from build123d import *

# Parameters (mm, degrees)
F0_W      = 210.82
F0_H      = 50.8
F1_DEPTH  = 12.7
F3_DEPTH  = 10.16
F4_DEPTH  = 3.175
F6_DEPTH  = 210.82
F7_DEPTH  = 5.5118
F8_SIZE2  = 5.499251
F8_SIZE   = 9.52499
F9_R      = 1.4605
F10_DEPTH = 9.525


# Not quite as in the source:
# - a fillet or chamfer is up to 0.001 mm smaller than in the source, because OpenCascade refuses the exact size


with BuildPart() as f1:
    # F0 (on Top) → F1 (new body)
    with BuildSketch(Plane.XY):
        with Locations((105.41, 25.4)):
            Rectangle(F0_W, F0_H)
    extrude(amount=F1_DEPTH)

    # F2 (on face) → F3 (cut)
    with BuildSketch(Plane.XY.offset(12.7)):
        with BuildLine():
            ThreePointArc((8.3320384182, 43.7379615818), (6.2559880613, 44.1509136731), (5.08, 42.3909231637))
            Line((5.08, 42.3909231637), (5.08, 8.4090768363))
            ThreePointArc((5.08, 8.4090768363), (6.2559880613, 6.6490863269), (8.3320384182, 7.0620384182))
            Line((8.3320384182, 7.0620384182), (25.3229615818, 24.0529615818))
            ThreePointArc((25.3229615818, 24.0529615818), (25.8809231637, 25.4), (25.3229615818, 26.7470384182))
            Line((25.3229615818, 26.7470384182), (8.3320384182, 43.7379615818))
        make_face()
        with BuildLine():
            Line((50.0879615818, 43.7379615818), (33.0970384182, 26.7470384182))
            ThreePointArc((33.0970384182, 26.7470384182), (32.5390768363, 25.4), (33.0970384182, 24.0529615818))
            Line((33.0970384182, 24.0529615818), (50.0879615818, 7.0620384182))
            ThreePointArc((50.0879615818, 7.0620384182), (52.1640119387, 6.6490863269), (53.34, 8.4090768363))
            Line((53.34, 8.4090768363), (53.34, 42.3909231637))
            ThreePointArc((53.34, 42.3909231637), (52.1640119387, 44.1509136731), (50.0879615818, 43.7379615818))
        make_face()
        with BuildLine():
            ThreePointArc((60.4020384182, 43.7379615818), (58.3259880613, 44.1509136731), (57.15, 42.3909231637))
            Line((57.15, 42.3909231637), (57.15, 8.4090768363))
            ThreePointArc((57.15, 8.4090768363), (58.3259880613, 6.6490863269), (60.4020384182, 7.0620384182))
            Line((60.4020384182, 7.0620384182), (77.3929615818, 24.0529615818))
            ThreePointArc((77.3929615818, 24.0529615818), (77.9509231637, 25.4), (77.3929615818, 26.7470384182))
            Line((77.3929615818, 26.7470384182), (60.4020384182, 43.7379615818))
        make_face()
        with BuildLine():
            Line((104.14, 8.4090768363), (104.14, 42.3909231637))
            ThreePointArc((104.14, 42.3909231637), (102.9640119387, 44.1509136731), (100.8879615818, 43.7379615818))
            Line((100.8879615818, 43.7379615818), (83.8970384182, 26.7470384182))
            ThreePointArc((83.8970384182, 26.7470384182), (83.3390768363, 25.4), (83.8970384182, 24.0529615818))
            Line((83.8970384182, 24.0529615818), (100.8879615818, 7.0620384182))
            ThreePointArc((100.8879615818, 7.0620384182), (102.9640119387, 6.6490863269), (104.14, 8.4090768363))
        make_face()
        with BuildLine():
            ThreePointArc((111.2020384182, 43.7379615818), (109.1259880613, 44.1509136731), (107.95, 42.3909231637))
            Line((107.95, 42.3909231637), (107.95, 8.4090768363))
            ThreePointArc((107.95, 8.4090768363), (109.1259880613, 6.6490863269), (111.2020384182, 7.0620384182))
            Line((111.2020384182, 7.0620384182), (128.1929615818, 24.0529615818))
            ThreePointArc((128.1929615818, 24.0529615818), (128.7509231637, 25.4), (128.1929615818, 26.7470384182))
            Line((128.1929615818, 26.7470384182), (111.2020384182, 43.7379615818))
        make_face()
        with BuildLine():
            Line((154.94, 8.4090768363), (154.94, 42.3909231637))
            ThreePointArc((154.94, 42.3909231637), (153.7640119387, 44.1509136731), (151.6879615818, 43.7379615818))
            Line((151.6879615818, 43.7379615818), (134.6970384182, 26.7470384182))
            ThreePointArc((134.6970384182, 26.7470384182), (134.1390768363, 25.4), (134.6970384182, 24.0529615818))
            Line((134.6970384182, 24.0529615818), (151.6879615818, 7.0620384182))
            ThreePointArc((151.6879615818, 7.0620384182), (153.7640119387, 6.6490863269), (154.94, 8.4090768363))
        make_face()
        with BuildLine():
            ThreePointArc((162.0020384182, 43.7379615818), (159.9259880613, 44.1509136731), (158.75, 42.3909231637))
            Line((158.75, 42.3909231637), (158.75, 8.4090768363))
            ThreePointArc((158.75, 8.4090768363), (159.9259880613, 6.6490863269), (162.0020384182, 7.0620384182))
            Line((162.0020384182, 7.0620384182), (178.9929615818, 24.0529615818))
            ThreePointArc((178.9929615818, 24.0529615818), (179.5509231637, 25.4), (178.9929615818, 26.7470384182))
            Line((178.9929615818, 26.7470384182), (162.0020384182, 43.7379615818))
        make_face()
        with BuildLine():
            Line((205.74, 8.4090768363), (205.74, 42.3909231637))
            ThreePointArc((205.74, 42.3909231637), (204.5640119387, 44.1509136731), (202.4879615818, 43.7379615818))
            Line((202.4879615818, 43.7379615818), (185.4970384182, 26.7470384182))
            ThreePointArc((185.4970384182, 26.7470384182), (184.9390768363, 25.4), (185.4970384182, 24.0529615818))
            Line((185.4970384182, 24.0529615818), (202.4879615818, 7.0620384182))
            ThreePointArc((202.4879615818, 7.0620384182), (204.5640119387, 6.6490863269), (205.74, 8.4090768363))
        make_face()
        with BuildLine():
            Line((44.9309231637, 46.99), (13.4890768363, 46.99))
            ThreePointArc((13.4890768363, 46.99), (11.7290863269, 45.8140119387), (12.1420384182, 43.7379615818))
            Line((12.1420384182, 43.7379615818), (27.8629615818, 28.0170384182))
            ThreePointArc((27.8629615818, 28.0170384182), (29.21, 27.4590768363), (30.5570384182, 28.0170384182))
            Line((30.5570384182, 28.0170384182), (46.2779615818, 43.7379615818))
            ThreePointArc((46.2779615818, 43.7379615818), (46.6909136731, 45.8140119387), (44.9309231637, 46.99))
        make_face()
        with BuildLine():
            ThreePointArc((12.1420384182, 7.0620384182), (11.7290863269, 4.9859880613), (13.4890768363, 3.81))
            Line((13.4890768363, 3.81), (44.9309231637, 3.81))
            ThreePointArc((44.9309231637, 3.81), (46.6909136731, 4.9859880613), (46.2779615818, 7.0620384182))
            Line((46.2779615818, 7.0620384182), (30.5570384182, 22.7829615818))
            ThreePointArc((30.5570384182, 22.7829615818), (29.21, 23.3409231637), (27.8629615818, 22.7829615818))
            Line((27.8629615818, 22.7829615818), (12.1420384182, 7.0620384182))
        make_face()
        with BuildLine():
            Line((95.7309231637, 46.99), (65.5590768363, 46.99))
            ThreePointArc((65.5590768363, 46.99), (63.7990863269, 45.8140119387), (64.2120384182, 43.7379615818))
            Line((64.2120384182, 43.7379615818), (79.2979615818, 28.6520384182))
            ThreePointArc((79.2979615818, 28.6520384182), (80.645, 28.0940768363), (81.9920384182, 28.6520384182))
            Line((81.9920384182, 28.6520384182), (97.0779615818, 43.7379615818))
            ThreePointArc((97.0779615818, 43.7379615818), (97.4909136731, 45.8140119387), (95.7309231637, 46.99))
        make_face()
        with BuildLine():
            ThreePointArc((64.2120384182, 7.0620384182), (63.7990863269, 4.9859880613), (65.5590768363, 3.81))
            Line((65.5590768363, 3.81), (95.7309231637, 3.81))
            ThreePointArc((95.7309231637, 3.81), (97.4909136731, 4.9859880613), (97.0779615818, 7.0620384182))
            Line((97.0779615818, 7.0620384182), (81.9920384182, 22.1479615818))
            ThreePointArc((81.9920384182, 22.1479615818), (80.645, 22.7059231637), (79.2979615818, 22.1479615818))
            Line((79.2979615818, 22.1479615818), (64.2120384182, 7.0620384182))
        make_face()
        with BuildLine():
            Line((146.5309231637, 46.99), (116.3590768363, 46.99))
            ThreePointArc((116.3590768363, 46.99), (114.5990863269, 45.8140119387), (115.0120384182, 43.7379615818))
            Line((115.0120384182, 43.7379615818), (130.0979615818, 28.6520384182))
            ThreePointArc((130.0979615818, 28.6520384182), (131.445, 28.0940768363), (132.7920384182, 28.6520384182))
            Line((132.7920384182, 28.6520384182), (147.8779615818, 43.7379615818))
            ThreePointArc((147.8779615818, 43.7379615818), (148.2909136731, 45.8140119387), (146.5309231637, 46.99))
        make_face()
        with BuildLine():
            ThreePointArc((115.0120384182, 7.0620384182), (114.5990863269, 4.9859880613), (116.3590768363, 3.81))
            Line((116.3590768363, 3.81), (146.5309231637, 3.81))
            ThreePointArc((146.5309231637, 3.81), (148.2909136731, 4.9859880613), (147.8779615818, 7.0620384182))
            Line((147.8779615818, 7.0620384182), (132.7920384182, 22.1479615818))
            ThreePointArc((132.7920384182, 22.1479615818), (131.445, 22.7059231637), (130.0979615818, 22.1479615818))
            Line((130.0979615818, 22.1479615818), (115.0120384182, 7.0620384182))
        make_face()
        with BuildLine():
            Line((197.3309231637, 46.99), (167.1590768363, 46.99))
            ThreePointArc((167.1590768363, 46.99), (165.3990863269, 45.8140119387), (165.8120384182, 43.7379615818))
            Line((165.8120384182, 43.7379615818), (180.8979615818, 28.6520384182))
            ThreePointArc((180.8979615818, 28.6520384182), (182.245, 28.0940768363), (183.5920384182, 28.6520384182))
            Line((183.5920384182, 28.6520384182), (198.6779615818, 43.7379615818))
            ThreePointArc((198.6779615818, 43.7379615818), (199.0909136731, 45.8140119387), (197.3309231637, 46.99))
        make_face()
        with BuildLine():
            ThreePointArc((165.8120384182, 7.0620384182), (165.3990863269, 4.9859880613), (167.1590768363, 3.81))
            Line((167.1590768363, 3.81), (197.3309231637, 3.81))
            ThreePointArc((197.3309231637, 3.81), (199.0909136731, 4.9859880613), (198.6779615818, 7.0620384182))
            Line((198.6779615818, 7.0620384182), (183.5920384182, 22.1479615818))
            ThreePointArc((183.5920384182, 22.1479615818), (182.245, 22.7059231637), (180.8979615818, 22.1479615818))
            Line((180.8979615818, 22.1479615818), (165.8120384182, 7.0620384182))
        make_face()
    extrude(amount=-F3_DEPTH, mode=Mode.SUBTRACT)

    # F4 (cut): a face of the model
    f4_faces = [f1.faces().sort_by_distance(p)[0] for p in [
        (105.41, 25.4, 0),
    ]]
    extrude(f4_faces, amount=-F4_DEPTH, mode=Mode.SUBTRACT)

    # F5 (on face) → F6 (join)
    with BuildSketch(Plane(origin=(0, 0, 0), x_dir=(0, -1, 0), z_dir=(-1, 0, 0))):
        Polygon((-56.299261314, 3.175), (-50.8, 3.175), (-50.8, 12.7), align=None)
        Polygon((0, 12.7), (0, 3.175), (5.499261314, 3.175), align=None)
    extrude(amount=-F6_DEPTH)

    # F7 (add): a face of the model
    f7_faces = [f1.faces().sort_by_distance(p)[0] for p in [
        (210.82, 25.4, 7.7824344249),
    ]]
    extrude(f7_faces, amount=F7_DEPTH)

    # F8 (size 9.525 and 5.499261314 in the source; OpenCascade refuses exactly that, so slightly less here)
    f8_edges = [f1.edges().sort_by_distance(p)[0] for p in [
        (216.3318, 25.4, 12.7),
    ]]
    f8_side = f1.faces().sort_by_distance((216.3318, 25.4, 7.782434))[0]
    chamfer(f8_edges, length=F8_SIZE, length2=F8_SIZE2, reference=f8_side)

    # F9 (on face) → F10 (cut)
    with BuildSketch(Plane.XY.offset(12.7)):
        with Locations((8.89, 46.99)):
            Circle(F9_R)
        with Locations((8.89, 3.81)):
            Circle(F9_R)
        with Locations((55.245, 46.99)):
            Circle(F9_R)
        with Locations((55.245, 3.81)):
            Circle(F9_R)
        with Locations((106.045, 46.99)):
            Circle(F9_R)
        with Locations((106.045, 3.81)):
            Circle(F9_R)
        with Locations((156.845, 46.99)):
            Circle(F9_R)
        with Locations((156.845, 3.81)):
            Circle(F9_R)
        with Locations((203.2, 46.99)):
            Circle(F9_R)
        with Locations((203.2, 3.81)):
            Circle(F9_R)
    extrude(amount=-F10_DEPTH, mode=Mode.SUBTRACT)


solid = f1.part
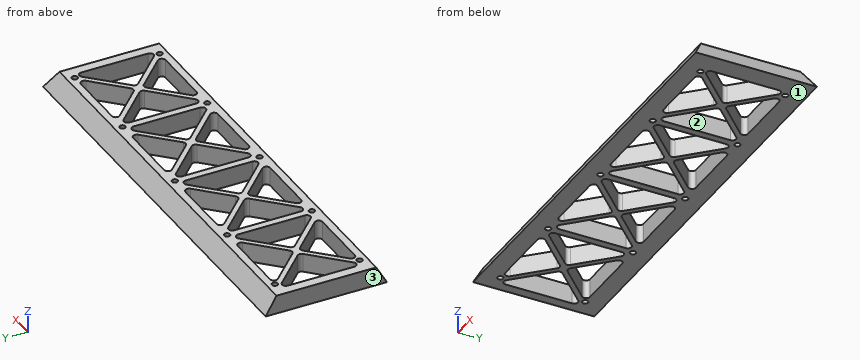
Design review of the part built by this model. Coordinates are the model's own, in mm. Face numbers are marked on the shaded views. Give positions to 0.01 mm unless a question says otherwise; leave off trailing zeros. Order: outer loops, then holes, each group sorted by start corner. A loop starts at its lowest first (then second) coordinate and runs counter-clockwise, first axis right, second up.
1. Add section B-B, the plane y = 40. State how many separate pieces and enclosed holes the cut face has, then the cut area to 3 significant figures.
Solution:
separate pieces: 13
enclosed holes: 0
area: 522 mm2
2. Add section A-A, the plane x = 37. State the section outline as (y, z) points (3 decimals), then the cut area to 3 significant figures.
Solution:
outline: (-5.499, 3.175) - (3.81, 3.175) - (3.81, 12.7) - (0, 12.7) - close; (16.34, 3.175) - (20.15, 3.175) - (20.15, 12.7) - (16.34, 12.7) - close; (30.65, 3.175) - (34.46, 3.175) - (34.46, 12.7) - (30.65, 12.7) - close; (46.99, 3.175) - (56.299, 3.175) - (50.8, 12.7) - (46.99, 12.7) - close
area: 198 mm2
3. Mouldability with a two-part tool opening along X and no side actions: class the marked faces 1, 2 and 3 as +X half, -X half, draft (parallel to the pull), parting line (faces both ways), or undercut.
Solution:
face 1: draft
face 2: undercut
face 3: -X half
4. For pin 1 Ø3.5 at (x, y) = (203.2, 46.99) entering from +Z; pin 2 Ø5 at (y, z) = (48.5, 6) entering from +X; pin 3 Ø3 at (x, z) = (133.5, 8) entering from -Y; pin 4 Ø1.8 at (x, y) = (8.89, 46.99) entering from -Z, all flat-tipped, find the tip position at first contact; note any pin that passes through.
Solution:
pin 1: stops at z = 12.7
pin 2: stops at x = 216.14
pin 3: stops at y = -3.58
pin 4: passes through
5. To check wall thickness, follow L1, parallel to Y at x = 203.2, z = 9; L2, parallel to Y at x = 8.89, z = 5.5; L3, parallel to Y at x = 112, z = 4.75. State the ranges of each line that lie inside material, in increasing order.
Solution:
L1: y = -2.14 to 2.35, 5.27 to 6.61, 44.19 to 45.53, 48.45 to 52.94
L2: y = -4.16 to 2.35, 5.27 to 7.62, 43.18 to 45.53, 48.45 to 54.96
L3: y = -4.59 to 7.86, 42.94 to 55.39
